Source: CAD feature listing. Evaluate the final solid. Frame: model axes, mm. Round coordinates to 2 decimals unless told otherwise and drop trailing zeros. Write each loop counter-clockwise with the first axis right and the second up, starting at its lowest first coordinate (ties: lowest second). Pieces come first, ordered by that corner, then holes.
from build123d import *

# Parameters (mm, degrees)
SKETCH1_W           = 429
SKETCH1_H           = 300
BOSS_EXTRUDE1_DEPTH = 10
SKETCH2_W           = 80
SKETCH2_H           = 160
SKETCH2_W_2         = 32
SKETCH2_H_2         = 98
SKETCH2_W_3         = 5
SKETCH2_H_3         = 24
CUT_EXTRUDE1_DEPTH  = 10


with BuildPart() as part:
    # Sketch1 → Boss-Extrude1 (new body)
    with BuildSketch(Plane(origin=(0, 0, 0), x_dir=(1, 0, 0), z_dir=(0, 1, 0))):
        Rectangle(SKETCH1_W, SKETCH1_H)
    extrude(amount=-BOSS_EXTRUDE1_DEPTH)

    # Sketch2 → Cut-Extrude1 (cut)
    with BuildSketch(Plane(origin=(0, 0, 0), x_dir=(1, 0, 0), z_dir=(0, 1, 0))):
        with Locations((-164.5, 60)):
            Rectangle(SKETCH2_W, SKETCH2_H)
        with Locations((-75.5, 60)):
            Rectangle(SKETCH2_W, SKETCH2_H)
        with Locations((13.5, 60)):
            Rectangle(SKETCH2_W, SKETCH2_H)
        Polygon((127.5, 140), (62.5, 140), (62.5, -3), (79.5, -3), (79.5, -52), (110.5, -52), (110.5, -3), (127.5, -3), align=None)
        with Locations((-146.5, -91)):
            Rectangle(SKETCH2_W_2, SKETCH2_H_2)
        with Locations((-188.5, -91)):
            Rectangle(SKETCH2_W_2, SKETCH2_H_2)
        with Locations((-104.5, -91)):
            Rectangle(SKETCH2_W_2, SKETCH2_H_2)
        with Locations((-62.5, -91)):
            Rectangle(SKETCH2_W_2, SKETCH2_H_2)
        with Locations((-20.5, -91)):
            Rectangle(SKETCH2_W_2, SKETCH2_H_2)
        with Locations((21.5, -91)):
            Rectangle(SKETCH2_W_2, SKETCH2_H_2)
        Polygon((153.5, -140), (184.5, -140), (184.5, -91), (201.5, -91), (201.5, 52), (136.5, 52), (136.5, -91), (153.5, -91), align=None)
        with Locations((-212, 129)):
            Rectangle(SKETCH2_W_3, SKETCH2_H_3)
        with Locations((212, -114)):
            Rectangle(SKETCH2_W_3, SKETCH2_H_3)
        with Locations((212, 129)):
            Rectangle(SKETCH2_W_3, SKETCH2_H_3)
        with Locations((-212, -112)):
            Rectangle(SKETCH2_W_3, SKETCH2_H_3)
    extrude(amount=-CUT_EXTRUDE1_DEPTH, mode=Mode.SUBTRACT)


solid = part.part
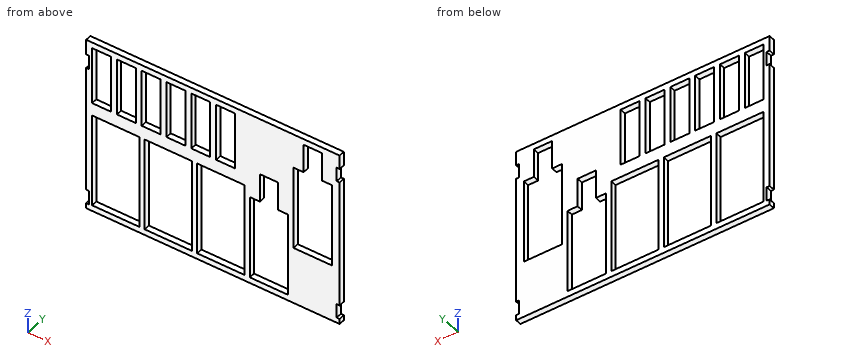
1) Material intervals for line 1 (X direction, y = -1.5, z = -123); line 2 (Z direction, x = -58.5, y = -7.25); line 3 (X direction, y = -4, z = 9), sorted ascending.
Taken from the geometry:
line 1: x = -209.5 to -204.5, -124.5 to -115.5, -35.5 to -26.5, 53.5 to 62.5, 127.5 to 209.5
line 2: z = -150 to -140, 20 to 42, 140 to 150
line 3: x = -214.5 to -204.5, -124.5 to -115.5, -35.5 to -26.5, 53.5 to 79.5, 110.5 to 136.5, 201.5 to 214.5
2) Section query D-D on x = 104. Return the cut outline in (y, z).
Taken from the geometry:
outline: (-10, -150) - (0, -150) - (0, -140) - (-10, -140) - close; (-10, 52) - (0, 52) - (0, 150) - (-10, 150) - close
3) Section query C-C on z = -22.5. Return the cut outline in (x, y), then the cut area to 3 significant figures.
Taken from the geometry:
outline: (-214.5, -10) - (-204.5, -10) - (-204.5, 0) - (-214.5, 0) - close; (-124.5, -10) - (-115.5, -10) - (-115.5, 0) - (-124.5, 0) - close; (-35.5, -10) - (-26.5, -10) - (-26.5, 0) - (-35.5, 0) - close; (53.5, -10) - (62.5, -10) - (62.5, 0) - (53.5, 0) - close; (127.5, -10) - (136.5, -10) - (136.5, 0) - (127.5, 0) - close; (201.5, -10) - (214.5, -10) - (214.5, 0) - (201.5, 0) - close
area: 590 mm2
4) Section query A-A on x = -183. Return the cut outline in (y, z).
Taken from the geometry:
outline: (-10, -150) - (0, -150) - (0, -140) - (-10, -140) - close; (-10, 20) - (0, 20) - (0, 42) - (-10, 42) - close; (-10, 140) - (0, 140) - (0, 150) - (-10, 150) - close
5) Section query B-B on z = 114.5. State how many separate pieces and enclosed holes the cut face has, then the cut area to 3 significant figures.
Taken from the geometry:
separate pieces: 8
enclosed holes: 0
area: 1,960 mm2
6) Contact query for a flat-ended pin moving along its axis: P1, Ø3, axis at y = -4, z = 108.5, coming from the +X side. Output: stop coordinate, or through.
Taken from the geometry:
P1: stops at x = 209.5
